from build123d import *

# Parameters (mm, degrees)
ESQUISSE1_W             = 36
ESQUISSE1_H             = 80
BOSS_EXTRU_1_DEPTH      = 3
ESQUISSE2_W             = 3
ESQUISSE2_H             = 55
BOSS_EXTRU_2_DEPTH      = 23
ESQUISSE3_W             = 3
ESQUISSE3_H             = 55
BOSS_EXTRU_3_DEPTH      = 33
ESQUISSE4_W             = 36
ESQUISSE4_H             = 25
ENL_V_MAT_EXTRU_1_DEPTH = 33


with BuildPart() as part:
    # Esquisse1 → Boss.-Extru.1 (new body)
    with BuildSketch(Plane.XY):
        with Locations((-27.15451692, 0.732402707)):
            Rectangle(ESQUISSE1_W, ESQUISSE1_H)
    extrude(amount=BOSS_EXTRU_1_DEPTH)

    # Esquisse2 → Boss.-Extru.2 (add)
    with BuildSketch(Plane(origin=(0, 0, 0), x_dir=(-1, 0, 0), z_dir=(0, 0, -1))):
        with Locations((10.65451692, 13.232402707)):
            Rectangle(ESQUISSE2_W, ESQUISSE2_H)
    extrude(amount=BOSS_EXTRU_2_DEPTH)

    # Esquisse3 → Boss.-Extru.3 (add)
    with BuildSketch(Plane.ZY.offset(12.15451692)):
        with Locations((-21.5, 13.232402707)):
            Rectangle(ESQUISSE3_W, ESQUISSE3_H)
    extrude(amount=BOSS_EXTRU_3_DEPTH)

    # Esquisse4 → Enlèv. mat.-Extru.1 (cut)
    with BuildSketch(Plane(origin=(0, 0, 0), x_dir=(-1, 0, 0), z_dir=(0, 0, -1))):
        with Locations((27.15451692, -26.767597293)):
            Rectangle(ESQUISSE4_W, ESQUISSE4_H)
    extrude(amount=-ENL_V_MAT_EXTRU_1_DEPTH, mode=Mode.SUBTRACT)


solid = part.part
The model under review builds one solid part; all positions refer to its coordinate system, in mm. A direction names the side the tool comes from. Give positions to 0.01 mm unless a question says otherwise; leave off trailing zeros. Loops run counter-clockwise (first coordinate to the right, second up) from the corner with the lowest first, then second, coordinate; pieces in that order, holes last. Notation, with made-up numbers: (-9.5, -5.5) -> (46.5, -5.5) arc R24 cw to (46.5, 21.5) -> close; hole circle Ø3 at (41, 77.5). An arc over 180 degrees is marked (long way). Put each result on its own line as item: value. Start each with the question number.
1. Mouldability with a two-part tool opening along Z and no side actions: class faces 3 (the face through (-27, 13, -23)), 4 (the face through (-12.155, 13, -10)), 5 (the face through (-9.155, 13, -10)), 6 (the face through (-28, 13, -20)) as released by +Z, released by -Z, zero draft, split by the parting line, or undercut.
2. We need section B-B on y = 13. State the section outline as (x, z) points.
3. We need section A-A on x = -28.5. State the section outline as (y, z) points, then the cut area to 3 significant figures.
4. We need section C-C on z = -4.75. State the section outline as (x, y) points, then the cut area to 3 significant figures.
5. Wall thickness on probe 1 along Z at (x, y) = (-36.5, 27); probe 2 along X at (y, z) = (36, -17): over which ranges is each line inside the solid? List them lowest first.
6. For faces 1 (the face through (-29, 14, 0)), 2 (the face through (-45.155, 14, -22)), list the 3-axis set-ups (+Z, -Z, +X, -X, +Y, -Y) from which the entire face can be reached by the end or side of a thin tool; tool diameter is ignored.
Determined:
1. face 3: released by -Z
1. face 4: undercut
1. face 5: zero draft
1. face 6: undercut
2. outline: (-45.15, -23) -> (-9.15, -23) -> (-9.15, 3) -> (-45.15, 3) -> (-45.15, 0) -> (-12.15, 0) -> (-12.15, -20) -> (-45.15, -20) -> close
3. outline: (-14.27, -23) -> (40.73, -23) -> (40.73, -20) -> (-14.27, -20) -> close; (-14.27, 0) -> (40.73, 0) -> (40.73, 3) -> (-14.27, 3) -> close
3. area: 330 mm^2
4. outline: (-12.15, -14.27) -> (-9.15, -14.27) -> (-9.15, 40.73) -> (-12.15, 40.73) -> close
4. area: 165 mm^2
5. probe 1: -23 to -20, 0 to 3
5. probe 2: -12.15 to -9.15
6. face 1: -X, +Y, -Y
6. face 2: +Z, -Z, -X, +Y, -Y
